Part model, mm, in its own coordinate system. Face numbers are marked on the shaded views. Coordinates: 2 decimals unless noted, no trailing zeros. Write each loop counter-clockwise with the first axis right and the second up, starting at its lowest first coordinate (ties: lowest second). Pieces come first, ordered by that corner, then holes. Notation, with made-up numbers: (16, 34) - (54, 34) arc R33 cw to (54, 73) - close; hole circle Ø11 at (20, 86). An arc over 180 degrees is marked (long way). Write each question's results on one line, items separated by ' | '.
from build123d import *

# Parameters (mm, degrees)
SKETCH021_W             = 51.5
SKETCH021_H             = 3
PAD014_DEPTH            = 1.6
SKETCH022_R             = 3
PAD015_DEPTH            = 2.6
HOLE_D                  = 3.4
HOLE_DEPTH              = 25
HOLE_CSINK_D            = 6.7
HOLE_CSINK_ANGLE        = 90
BODY005_PLACEMENT_ANGLE = 180


with BuildPart() as part:
    # Sketch021 → Pad014 (new body)
    with BuildSketch(Plane.XY):
        with BuildLine():
            ThreePointArc((-44, 40), (-47.535534, 38.535534), (-49, 35))
            Line((-49, -35), (-49, 35))
            ThreePointArc((-49, -35), (-47.535534, -38.535534), (-44, -40))
            Line((44, -40), (-44, -40))
            ThreePointArc((44, -40), (47.535534, -38.535534), (49, -35))
            Line((49, 35), (49, -35))
            ThreePointArc((49, 35), (47.535534, 38.535534), (44, 40))
            Line((-44, 40), (44, 40))
        make_face()
        with Locations((0, 21.5)):
            Rectangle(SKETCH021_W, SKETCH021_H, mode=Mode.SUBTRACT)
        with Locations((0, -21.5)):
            Rectangle(SKETCH021_W, SKETCH021_H, mode=Mode.SUBTRACT)
    extrude(amount=PAD014_DEPTH)

    # Sketch022 → Pad015 (join)
    with BuildSketch(Plane.XY):
        with Locations((-45, 36)):
            Circle(SKETCH022_R)
        with Locations((11, 36)):
            Circle(SKETCH022_R)
        with Locations((45, 36)):
            Circle(SKETCH022_R)
        with Locations((45, -36)):
            Circle(SKETCH022_R)
        with Locations((11, -36)):
            Circle(SKETCH022_R)
        with Locations((-45, -36)):
            Circle(SKETCH022_R)
    extrude(amount=PAD015_DEPTH)

    # Hole
    with Locations(Plane(origin=(0, 0, 0), x_dir=(1, 0, 0), z_dir=(0, 0, -1))):
        with Locations((-45, -36), (11, -36), (45, -36), (45, 36), (11, 36), (-45, 36)):
            CounterSinkHole(HOLE_D / 2, HOLE_CSINK_D / 2, depth=HOLE_DEPTH, counter_sink_angle=HOLE_CSINK_ANGLE)


with BuildPart() as part_1:
    # Body005 placement: moved
    add(part.part.moved(Location((0, 0, 80.3))).rotate(Axis((0, 0, 80.3), (1, 0, 0)), BODY005_PLACEMENT_ANGLE))


solid = part_1.part
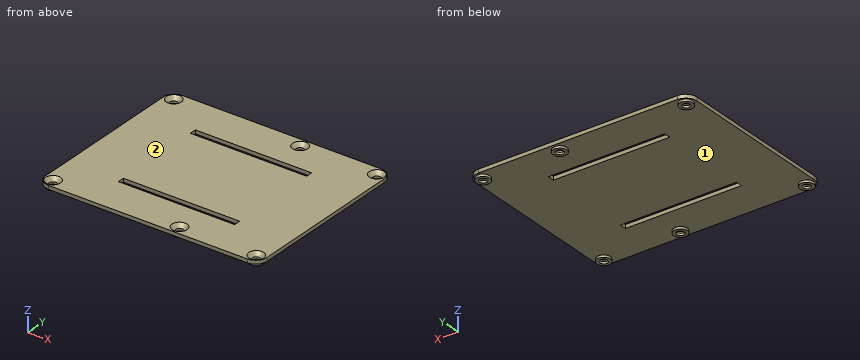
(1) Two-plate mould, pull along Y, no slides. Class the marked faces 1 and 2: released by +Y, released by -Y, zero draft, split by the parting line, or undercut.
Return value:
face 1: undercut | face 2: zero draft
(2) Wall check: line 1 (X direction, y = 36, z = 77.95); line 2 (Y direction, x = -45, z = 78); line 3 (Y direction, x = 3, z = 79.5). Give the ranges that are in metal, low to high. Write a range as from..to.
Return value:
line 1: x = -48..-46.7, -43.3..-42, 8..9.3, 12.7..14, 42..43.3, 46.7..48 | line 2: y = -39..-37.7, -34.3..-33, 33..34.3, 37.7..39 | line 3: y = -40..-23, -20..20, 23..40
(3) Saw through at A-A on z = 78.15. Count the separate pieces of the cut face and the enclosed holes in it, then the cut area to 3 significant figures.
Return value:
separate pieces: 6 | enclosed holes: 6 | area: 115 mm^2
(4) Saw through at C-C on x = -8. Write the cut outline in (y, z), then the cut area to 3 significant figures.
Return value:
outline: (-40, 78.7) - (-23, 78.7) - (-23, 80.3) - (-40, 80.3) - close; (-20, 78.7) - (20, 78.7) - (20, 80.3) - (-20, 80.3) - close; (23, 78.7) - (40, 78.7) - (40, 80.3) - (23, 80.3) - close | area: 118 mm^2
(5) Saw through at D-D on y = 8. Write the cut outline in (x, z).
Return value:
outline: (-49, 78.7) - (49, 78.7) - (49, 80.3) - (-49, 80.3) - close
